Here's how the part is built. I have some questions about the finished solid (model axes, mm). Face numbers are marked on the shaded views. A direction names the side the tool comes from. Round coordinates to 2 decimals unless told otherwise and drop trailing zeros. Loops run counter-clockwise (first coordinate to the right, second up) from the corner with the lowest first, then second, coordinate; pieces in that order, holes last. Notation, with made-up numbers: (33, 7) -> (71, 7) arc R23 ccw to (71, 18) -> close; hole circle Ø2 at (60, 56.5). An arc over 180 degrees is marked (long way). Use one line per item in the form item = value. Start each with the question number.
Item 1: If we section it at C-C (y = 15): Write out the boundary of the cut face in (x, z).
Item 2: I'm going to push flat-ended pins straight in: pin 1 Ø12 at (x, y) = (-57, -9.5) entering from +Z; pin 2 Ø3 at (y, z) = (13, 18) entering from +X; pin 3 Ø13 at (x, y) = (-57, 0) entering from +Z; pin 4 Ø8 at (x, z) = (60, 8.5) entering from +Y. Where does each tip first touch, or does it pass through?
Item 3: If we section it at B-B (z = 31): Write out the boundary of the cut face in (x, y).
Item 4: For the marked faces 4, 5, 6 and 7, which set-ups out of +Z, -Z, +X, -X, +Y, -Y let a thin tool reach every point of the face, with its end or its side?
Item 5: If I drill on L1, parallel to X at y = 0, z = 6.5; L2, parallel to Y at x = -57, z = 10; L3, parallel to X at y = -21, z = 51, over which ranges is the centre line in solid material (lowest first)? Write a range as [from, to].
Item 6: If we section it at D-D (z = 24): Write out the boundary of the cut face in (x, y).
Item 7: If we section it at A-A (z = 4.5): State how many separate pieces and enclosed holes the cut face has, then the cut area to 3 significant figures.
Item 8: Thinking about a two-plate mould opening in X: for the marked faces 1, 2 and 3, which applies, released by +X, released by -X, zero draft, split by the parting line, or undercut?
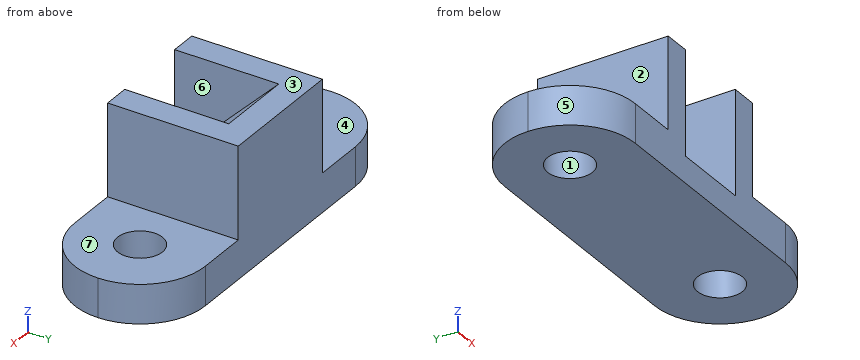
Autodesk Fusion 360 part; units mm, degrees
sketch "base" plane through (0, 0, 0) normal (0, 0, 1) x (1, 0, 0)
  line L0 (89, 32) -> (-89, 32)
  line L1 (-89, 32) -> (-89, -32)
  line L2 (-89, -32) -> (89, -32)
  line L3 (89, -32) -> (89, 32)
  line L4 (89, 32) -> (-89, -32) construction
  line L5 (-89, 32) -> (89, -32) construction
  dimension "d1" = 178
  dimension "d2" = 64
extrude "Extrude1" add sketch "base" along normal blind 19
fillet "Fillet1" radius 32 4 edges at (89, -32, 9.5) (89, 32, 9.5) (-89, -32, 9.5) (-89, 32, 9.5)
sketch "circles" plane through (0, 0, 19) normal (0, 0, 1) x (-1, 0, 0)
  arc A0 (57, -32) -> (57, 32) centre (57, 0) ccw
  line L0 (57, 32) -> (-57, 32)
  arc A1 (-57, 32) -> (-57, -32) centre (-57, 0) ccw
  line L1 (-57, -32) -> (57, -32)
  line L2 (57, 32) -> (57, -32) construction
  line L3 (-57, 32) -> (-57, -32) construction
  circle A2 centre (-57, 0) radius 11
  circle A3 centre (57, 0) radius 11
  dimension "d6" = 64
  dimension "d7" = 64
  dimension "d8" = 22
  dimension "d9" = 22
extrude "Extrude2" cut sketch "circles" against normal blind 50 contours A2 | A3
sketch "base square" plane through (0, 0, 19) normal (0, 0, 1) x (-1, 0, 0)
  circle A0 centre (57, 0) radius 11
  circle A1 centre (-57, 0) radius 11
  arc A2 (57, -32) -> (57, 32) centre (57, 0) ccw
  line L0 (57, 32) -> (-57, 32)
  arc A3 (-57, 32) -> (-57, -32) centre (-57, 0) ccw
  line L1 (-57, -32) -> (57, -32)
  line L2 (-32, -32) -> (32, -32)
  line L3 (32, -32) -> (32, 32)
  line L4 (32, 32) -> (-32, 32)
  line L5 (-32, 32) -> (-32, -32)
  line L6 (-32, -32) -> (32, 32) construction
  line L7 (32, -32) -> (-32, 32) construction
  dimension "d12" = 64
  dimension "d13" = 64
extrude "Extrude3" add sketch "base square" along normal blind 45 contours L0 L1 L2 L3 L4 L5
sketch "top rectangle" plane through (0, 0, 64) normal (0, 0, 1) x (-1, 0, 0)
  line L0 (-32, 32) -> (-32, -32)
  line L1 (-32, -32) -> (32, -32)
  line L2 (32, -32) -> (32, 32)
  line L3 (32, 32) -> (-32, 32)
  line L4 (19, 32) -> (-19, 32)
  line L5 (-19, 32) -> (-19, -19)
  line L6 (-19, -19) -> (19, -19)
  line L7 (19, -19) -> (19, 32)
  dimension "d16" = 13
  dimension "d17" = 38
  dimension "d18" = 51
extrude "Extrude4" cut sketch "top rectangle" against normal blind 51 contours L3 L4 L5 L6 L7
sketch "Sketch6" plane through (-19, 0, 0) normal (1, 0, 0) x (0, 1, 0)
  line L0 (19, 64) -> (-32, 64)
  line L1 (-32, 64) -> (-32, 13)
  line L2 (-32, 13) -> (19, 13)
  line L3 (19, 13) -> (19, 64)
  line L4 (-32, 13) -> (19, 13)
  line L5 (19, 13) -> (19, 64)
  line L6 (-32, 13) -> (19, 64)
extrude "Extrude5" add sketch "Sketch6" along normal blind 38 contours L2 L3 L4 L5 L6
equation "d1 = 114 mm + 32 mm + 32 mm"
equation "d14 = 64 mm - 19 mm"
equation "d19 = -64 mm + 19 mm - 6 mm"
Values found:
q1.outline = (-85.27, 0) -> (85.27, 0) -> (85.27, 19) -> (32, 19) -> (32, 64) -> (19, 64) -> (19, 60) -> (-19, 60) -> (-19, 64) -> (-32, 64) -> (-32, 19) -> (-85.27, 19) -> close
q2.pin_1 = 19
q2.pin_2 = 86.86
q2.pin_3 = through
q2.pin_4 = 32
q3.outline = (-32, -32) -> (-19, -32) -> (-19, -14) -> (19, -14) -> (19, -32) -> (32, -32) -> (32, 32) -> (-32, 32) -> close
q4.face_4 = +Z, -X, +Y, -Y
q4.face_5 = +Z, -Z, -X, -Y
q4.face_6 = +Z, -Y
q4.face_7 = +Z, +X, +Y, -Y
q5.L1 = [-89, -68], [-46, 46], [68, 89]
q5.L2 = [-32, -11], [11, 32]
q5.L3 = [-32, -19], [19, 32]
q6.outline = (-32, -32) -> (-19, -32) -> (-19, -21) -> (19, -21) -> (19, -32) -> (32, -32) -> (32, 32) -> (-32, 32) -> close
q7.separate_pieces = 1
q7.enclosed_holes = 2
q7.area = 9,750 mm2
q8.face_1 = undercut
q8.face_2 = released by -X
q8.face_3 = zero draft
